The model under review builds one solid part; all positions refer to its coordinate system, in mm. A direction names the side the tool comes from. Coordinates: 2 decimals unless noted, no trailing zeros. Write each loop counter-clockwise with the first axis right and the second up, starting at its lowest first coordinate (ties: lowest second). Pieces come first, ordered by that corner, then holes.
1) For line 1 (Y direction, x = 25.5, z = -0.75); line 2 (X direction, y = -11.5, z = 2.25); line 3 (Y direction, x = 21, z = 4.5), list the stretches that pass through material, from the lowest coordinate up.
2) Add section C-C, the plane z = -2. State the section outline as (x, y) points, then the cut area to 3 significant figures.
3) Mouldability with a two-part tool opening along X and no side actions: class faces 4 (the flat face through (0, 1, 7)), 5 (the cylindrical face through (31.15, 0.72, 6.43)), 6 (the flat face through (-29, 4.75, 1)) as released by +X, released by -X, zero draft, split by the parting line, or undercut.
4) Machinability: for faces 1 (the flat face through (-29, 4.75, 4)), 2 (the flat face through (-24, -9.25, 6)), 3 (the flat face through (0, -16.5, -1)), which of the approach directions +Z, -Z, +X, -X, +Y, -Y give a long, thin tool a straight path to every point of the face, cutting with its end or side? Answer none if there is none.
5) For P1, Ø1.5, axis at x = 13.5, y = -12.5, coming from the -Z side; P2, Ø0.5, axis at y = 8.5, z = 6.5, coming from the +X side; P3, Ø0.8, axis at x = -24, z = 6, coming from the -Y side, all flat-tipped, find the tip position at first contact; note any pin that passes through.
6) Add section A-A, the plane y = 1. State the section outline as (x, z) points, then the cut area to 3 significant figures.
7) Add section B-B, the plane x = 10.5. State the section outline as (y, z) points, then the cut area to 3 significant figures.
8) Add section D-D, the plane x = -10.5. State the section outline as (y, z) points.
from build123d import *

# Parameters (mm, degrees)
F0_W          = 62.5
F0_H          = 36.5
F0_W_2        = 58.5
F0_H_2        = 31.5
F1_DEPTH      = 7
F2_W          = 4
F2_H          = 3
F3_DEPTH      = 1.5
F4_W          = 62.5
F4_H          = 36.5
F5_DEPTH      = 3
F7_DEPTH      = 2.5
F8_R          = 2.5
F9_R          = 1
F10_R         = 1
F11_T1_DEPTH  = 57.5
F11_T3_DEPTH  = 31.5
F11_T6_ANGLE  = 90
F11_T8_ANGLE  = 90
F11_T10_ANGLE = 90
F11_T12_ANGLE = 90
F12_W         = 1.25
F12_H         = 8.5
F13_DEPTH     = 2


# Not quite as in the source:
# - a fillet or chamfer that OpenCascade refuses, or shapes differently, is made with other operations: its cross-section is extruded or revolved along the edge and cut away or added


with BuildPart() as f1:
    # F0 (on Top) → F1 (new body)
    with BuildSketch(Plane.XY):
        with Locations((0.5, 0.5)):
            Rectangle(F0_W, F0_H)
        with Locations((1, 0.5)):
            Rectangle(F0_W_2, F0_H_2, mode=Mode.SUBTRACT)
    extrude(amount=F1_DEPTH)

    # F2 (on face) → F3 (join)
    with BuildSketch(Plane.XY.offset(7)):
        Polygon((30.25, 16.25), (-28.25, 16.25), (-28.25, -15.25), (30.25, -15.25), (30.25, -6), (5.25, -6), (5.25, 7), (30.25, 7), align=None)
        with Locations((-24.25, -7.75)):
            Rectangle(F2_W, F2_H, mode=Mode.SUBTRACT)
        with Locations((-24.25, 8.75)):
            Rectangle(F2_W, F2_H, mode=Mode.SUBTRACT)
    extrude(amount=-F3_DEPTH)

    # F4 (on face) → F5 (join)
    with BuildSketch(Plane(origin=(0, 0, 0), x_dir=(1, 0, 0), z_dir=(0, 0, -1))):
        with Locations((0.5, -0.5)):
            Rectangle(F4_W, F4_H)
        Polygon((-29.5, -17.522141248), (-29.5, 16.5), (30.25, 16.5), (30.25, 15.25), (30.25, -16.25), (30.25, -17.522141248), align=None, mode=Mode.SUBTRACT)
    extrude(amount=F5_DEPTH)

    # F6 (on face) → F7 (cut)
    with BuildSketch(Plane.YZ.offset(-28.25)):
        with BuildLine():
            Line((4, 5.5), (-3, 5.5))
            ThreePointArc((-3, 5.5), (-3.5303300859, 5.2803300859), (-3.75, 4.75))
            Line((-3.75, 4.75), (-3.75, 3.5))
            ThreePointArc((-3.75, 3.5), (-3.1642135624, 2.0857864376), (-1.75, 1.5))
            Line((-1.75, 1.5), (2.75, 1.5))
            ThreePointArc((2.75, 1.5), (4.1642135624, 2.0857864376), (4.75, 3.5))
            Line((4.75, 3.5), (4.75, 4.75))
            ThreePointArc((4.75, 4.75), (4.5303300859, 5.2803300859), (4, 5.5))
        make_face()
    extrude(amount=-F7_DEPTH, mode=Mode.SUBTRACT)

    # F8
    f8_edges = [f1.edges().sort_by_distance(p)[0] for p in [
        (-30.75, 18.75, 2),
        (-30.75, -17.75, 2),
        (31.75, 18.75, 2),
        (31.75, -17.75, 2),
    ]]
    fillet(f8_edges, radius=F8_R)

    # F9
    f9_edges = [f1.edges().sort_by_distance(p)[0] for p in [
        (5.25, 7, 6.25),
        (30.25, 7, 6.25),
        (30.25, -6, 6.25),
        (5.25, -6, 6.25),
    ]]
    fillet(f9_edges, radius=F9_R)

    # F10
    f10_edges = [f1.edges().sort_by_distance(p)[0] for p in [
        (-22.25, 10.25, 6.25),
        (-26.25, 10.25, 6.25),
        (-26.25, 7.25, 6.25),
        (-22.25, 7.25, 6.25),
        (-26.25, -6.25, 6.25),
        (-22.25, -6.25, 6.25),
        (-22.25, -9.25, 6.25),
        (-26.25, -9.25, 6.25),
    ]]
    fillet(f10_edges, radius=F10_R)

    # F11: fillet of radius 2 on 8 edges, made by hand

    # F11_s2 → F11_t1 (cut)
    with BuildSketch(Plane.YZ.offset(-28.25)):
        with BuildLine():
            ThreePointArc((-15.75, 7), (-17.1642135624, 6.4142135624), (-17.75, 5))
            Line((-17.75, 5), (-17.75, 7))
            Line((-17.75, 7), (-15.75, 7))
        make_face()
        with BuildLine():
            ThreePointArc((16.75, 7), (18.1642135624, 6.4142135624), (18.75, 5))
            Line((18.75, 5), (18.75, 7))
            Line((18.75, 7), (16.75, 7))
        make_face()
    extrude(amount=F11_T1_DEPTH, mode=Mode.SUBTRACT)

    # F11_s4 → F11_t3 (cut)
    with BuildSketch(Plane.XZ.offset(-16.25)):
        with BuildLine():
            ThreePointArc((29.75, 7), (31.1642135624, 6.4142135624), (31.75, 5))
            Line((31.75, 5), (31.75, 7))
            Line((31.75, 7), (29.75, 7))
        make_face()
        with BuildLine():
            ThreePointArc((-28.75, 7), (-30.1642135624, 6.4142135624), (-30.75, 5))
            Line((-30.75, 5), (-30.75, 7))
            Line((-30.75, 7), (-28.75, 7))
        make_face()
    extrude(amount=F11_T3_DEPTH, mode=Mode.SUBTRACT)

    # F11_s5 → F11_t6 (revolve, cut)
    with BuildSketch(Plane.YZ.offset(29.25)):
        with BuildLine():
            ThreePointArc((16.75, 7), (18.1642135624, 6.4142135624), (18.75, 5))
            Line((18.75, 5), (18.75, 7))
            Line((18.75, 7), (16.75, 7))
        make_face()
    revolve(axis=Axis((29.25, 16.25, 7), (0, 0, -1)), revolution_arc=F11_T6_ANGLE, mode=Mode.SUBTRACT)

    # F11_s7 → F11_t8 (revolve, cut)
    with BuildSketch(Plane.YZ.offset(-28.25)):
        with BuildLine():
            ThreePointArc((16.75, 7), (18.1642135624, 6.4142135624), (18.75, 5))
            Line((18.75, 5), (18.75, 7))
            Line((18.75, 7), (16.75, 7))
        make_face()
    revolve(axis=Axis((-28.25, 16.25, 7), (0, 0, 1)), revolution_arc=F11_T8_ANGLE, mode=Mode.SUBTRACT)

    # F11_s9 → F11_t10 (revolve, cut)
    with BuildSketch(Plane.XZ.offset(15.25)):
        with BuildLine():
            ThreePointArc((29.75, 7), (31.1642135624, 6.4142135624), (31.75, 5))
            Line((31.75, 5), (31.75, 7))
            Line((31.75, 7), (29.75, 7))
        make_face()
    revolve(axis=Axis((29.25, -15.25, 7), (0, 0, -1)), revolution_arc=F11_T10_ANGLE, mode=Mode.SUBTRACT)

    # F11_s11 → F11_t12 (revolve, cut)
    with BuildSketch(Plane.XZ.offset(15.25)):
        with BuildLine():
            ThreePointArc((-28.75, 7), (-30.1642135624, 6.4142135624), (-30.75, 5))
            Line((-30.75, 5), (-30.75, 7))
            Line((-30.75, 7), (-28.75, 7))
        make_face()
    revolve(axis=Axis((-28.25, -15.25, 7), (0, 0, 1)), revolution_arc=F11_T12_ANGLE, mode=Mode.SUBTRACT)

    # F12 (on face) → F13 (cut)
    with BuildSketch(Plane(origin=(0, 0, 0), x_dir=(1, 0, 0), z_dir=(0, 0, -1))):
        with Locations((-28.875, -0.5)):
            Rectangle(F12_W, F12_H)
    extrude(amount=-F13_DEPTH, mode=Mode.SUBTRACT)


solid = f1.part
Geometry results:
1. line 1: y = -17.75 to -16.5, 17.52 to 18.75
1. line 2: x = -30.75 to -28.25, 30.25 to 31.75
1. line 3: y = -17.75 to -15.25, 16.25 to 18.75
2. outline: (-30.75, -15.25) arc R2.5 ccw to (-28.25, -17.75) - (29.25, -17.75) arc R2.5 ccw to (31.75, -15.25) - (31.75, 16.25) arc R2.5 ccw to (29.25, 18.75) - (-28.25, 18.75) arc R2.5 ccw to (-30.75, 16.25) - close; hole (-29.5, -16.5) - (30.25, -16.5) - (30.25, 17.52) - (-29.5, 17.52) - close
2. area: 243 mm2
3. face 4: zero draft
3. face 5: released by +X
3. face 6: undercut
4. face 1: -X
4. face 2: +Z, -Z
4. face 3: -Z
5. P1: stops at z = 5.5
5. P2: stops at x = 31.31
5. P3: stops at y = -17.66
6. outline: (-30.75, -3) - (-29.5, -3) - (-29.5, 1.5) - (-30.75, 1.5) - close; (-30.69, 5.5) - (5.25, 5.5) - (5.25, 7) - (-28.75, 7) arc R2 ccw to start; (30.25, -3) - (31.75, -3) - (31.75, 5) arc R2 ccw to (30.25, 6.94) - close
6. area: 72.9 mm2
7. outline: (-17.75, -3) - (-16.5, -3) - (-16.5, 0) - (-15.25, 0) - (-15.25, 5.5) - (-6, 5.5) - (-6, 7) - (-15.75, 7) arc R2 ccw to (-17.75, 5) - close; (7, 5.5) - (16.25, 5.5) - (16.25, 0) - (17.52, 0) - (17.52, -3) - (18.75, -3) - (18.75, 5) arc R2 ccw to (16.75, 7) - (7, 7) - close
7. area: 68.5 mm2
8. outline: (-17.75, -3) - (-16.5, -3) - (-16.5, 0) - (-15.25, 0) - (-15.25, 5.5) - (16.25, 5.5) - (16.25, 0) - (17.52, 0) - (17.52, -3) - (18.75, -3) - (18.75, 5) arc R2 ccw to (16.75, 7) - (-15.75, 7) arc R2 ccw to (-17.75, 5) - close
